Could you check a few things on this model? Use its own coordinates, in mm. A direction names the side the tool comes from. Round coordinates to 2 decimals unless told otherwise and drop trailing zeros. Write each loop counter-clockwise with the first axis right and the second up, starting at its lowest first coordinate (ties: lowest second). Pieces come first, ordered by that corner, then holes. Notation, with made-up numbers: (33, 73.25) -> (87, 73.25) arc R24 ccw to (87, 108.25) -> close; hole circle Ø5 at (36.25, -33). An arc over 180 degrees is marked (long way). Answer as CSV lines item,"result". Start each with the question number.
Q1. Imagine slicing it at D-D on z = 28.5. Please give me the cut outline in (x, y), and give its area (3 significant figures).
Q2. Imagine slicing it at C-C on x = -15. Please give me the cut outline in (y, z), and give its area (3 significant figures).
Q3. If I drill on line 1 (Y direction, x = 26, z = 9); line 2 (Y direction, x = -32.5, z = 38.5); line 3 (X direction, y = 37, z = 56), over which ranges is the centre line in solid material (lowest first)? Write a range as [from, to].
Q4. Will these pins go through, and if not, where does the flat tip stop? pin 1 Ø10 at (x, z) = (-39.5, 44.5) entering from -Y; pin 2 Ø8 at (x, z) = (-22, 10) entering from +Y; pin 3 Ø4 at (x, y) = (39.5, -3.5) entering from +Z.
Q5. Imagine slicing it at A-A on z = 49. Please give me the cut outline in (x, y).
Q6. Imagine slicing it at B-B on y = 22.5. Please give me the cut outline in (x, z).
Q7. If we mould it in two halves opening along Y, with no side actions, what happens to faces 4 (the flat face through (-27, -1, 63.5)), 5 (the flat face through (1, 29.04, 31)), 6 (the cylindrical face through (42.595, -4.481, 50.978))? For each: pulls with the +Y half, pulls with the -Y half, needs draft (parallel to the pull), parting line crosses it, or undercut.
Q8. For faces 1 (the flat face through (-34, -2, 38.1)), 2 (the cylindrical face through (0.95, 38.05, 40.91)), 3 (the flat face through (1, -33.137, 31)), which set-ups out of +Z, -Z, +X, -X, +Y, -Y let a thin tool reach every point of the face, with its end or its side?
from build123d import *

# Parameters (mm, degrees)
F0_W      = 108.688287437
F0_H      = 62.1764454991
F1_DEPTH  = 63.5
F2_R      = 6.35
F3_DEPTH  = 25.4
F4_W      = 45.188287437
F4_H      = 17.78
F4_H_2    = 62.1764454991
F5_DEPTH  = 25.4
F7_DEPTH  = 17.78
F9_DEPTH  = 97.7364454991
F11_DEPTH = 17.78
F13_DEPTH = 17.78


with BuildPart() as f1:
    # F0 (on Top) → F1 (new body)
    with BuildSketch(Plane.XY):
        with Locations((1.4459639788, -2.0484467968)):
            Rectangle(F0_W, F0_H)
    extrude(amount=F1_DEPTH)

    # F2 (on face) → F3 (cut)
    with BuildSketch(Plane.XY.offset(63.5)):
        with Locations((-33.8375324716, -2.0484467968)):
            Circle(F2_R)
        with Locations((36.7294604292, -2.0484467968)):
            Circle(F2_R)
    extrude(amount=-F3_DEPTH, mode=Mode.SUBTRACT)

    # F4 (on face) → F5 (join)
    with BuildSketch(Plane.XY.offset(63.5)):
        with Locations((1.4459639788, -42.0266695464)):
            Rectangle(F4_W, F4_H)
        with Locations((1.4459639788, -2.0484467968)):
            Rectangle(F4_W, F4_H_2)
        with Locations((1.4459639788, 37.9297759527)):
            Rectangle(F4_W, F4_H)
    extrude(amount=-F5_DEPTH)

    # F6 (on face) → F7 (cut, through all)
    with BuildSketch(Plane.XZ.offset(50.9166695464)):
        with BuildLine():
            ThreePointArc((24.0401076972, 63.5), (1.4459639788, 40.9058562815), (-21.1481797397, 63.5))
            Line((-21.1481797397, 63.5), (-21.1481797397, 38.1))
            Line((-21.1481797397, 38.1), (24.0401076972, 38.1))
            Line((24.0401076972, 38.1), (24.0401076972, 63.5))
        make_face()
    extrude(amount=-F7_DEPTH, mode=Mode.SUBTRACT)

    # F8 (on face) → F9 (cut, through all)
    with BuildSketch(Plane.XZ.offset(50.9166695464)):
        with BuildLine():
            Line((20.2301076972, 63.5), (-17.3381797397, 63.5))
            ThreePointArc((-17.3381797397, 63.5), (1.4459639788, 45.134926003), (20.2301076972, 63.5))
        make_face()
    extrude(amount=-F9_DEPTH, mode=Mode.SUBTRACT)

    # F10 (on face) → F11 (join, through all)
    with BuildSketch(Plane(origin=(0, 46.8197759527, 0), x_dir=(-1, 0, 0), z_dir=(0, 1, 0))):
        with BuildLine():
            ThreePointArc((21.1481797397, 63.5), (-1.4459639788, 40.9058562815), (-24.0401076972, 63.5))
            Line((-24.0401076972, 63.5), (-24.0401076972, 38.1))
            Line((-24.0401076972, 38.1), (21.1481797397, 38.1))
            Line((21.1481797397, 38.1), (21.1481797397, 63.5))
        make_face()
    extrude(amount=-F11_DEPTH)

    # F12 (on face) → F13 (cut, through all)
    with BuildSketch(Plane(origin=(0, 46.8197759527, 0), x_dir=(-1, 0, 0), z_dir=(0, 1, 0))):
        with BuildLine():
            ThreePointArc((21.1481797397, 63.5), (-1.4459639788, 40.9058562815), (-24.0401076972, 63.5))
            Line((-24.0401076972, 63.5), (-24.0401076972, 38.1))
            Line((-24.0401076972, 38.1), (21.1481797397, 38.1))
            Line((21.1481797397, 38.1), (21.1481797397, 63.5))
        make_face()
    extrude(amount=-F13_DEPTH, mode=Mode.SUBTRACT)


solid = f1.part
Checks:
1,outline,"(-52.9, -33.14) -> (55.79, -33.14) -> (55.79, 29.04) -> (-52.9, 29.04) -> close"
1,area,"6,760 mm^2"
2,outline,"(-50.92, 48.01) -> (-33.14, 48.01) -> (-33.14, 0) -> (29.04, 0) -> (29.04, 48.01) -> (46.82, 48.01) -> (46.82, 54.84) -> (-50.92, 54.84) -> close"
2,area,"3,650 mm^2"
3,line 1,"[-33.14, 29.04]"
3,line 2,"[-33.14, -8.26], [4.16, 29.04]"
3,line 3,"[-19.87, -15.59], [18.48, 22.76]"
4,pin 1,"y = -33.14"
4,pin 2,"y = 29.04"
4,pin 3,"z = 38.1"
5,outline,"(-52.9, -33.14) -> (-15.88, -33.14) -> (-15.88, -50.92) -> (-9.97, -50.92) -> (-9.97, 46.82) -> (-15.88, 46.82) -> (-15.88, 29.04) -> (-52.9, 29.04) -> close; (12.86, -50.92) -> (18.77, -50.92) -> (18.77, -33.14) -> (55.79, -33.14) -> (55.79, 29.04) -> (18.77, 29.04) -> (18.77, 46.82) -> (12.86, 46.82) -> close; hole circle Ø12.7 at (-33.84, -2.05); hole circle Ø12.7 at (36.73, -2.05)"
6,outline,"(-52.9, 0) -> (55.79, 0) -> (55.79, 63.5) -> (20.23, 63.5) arc R18.79 cw to (-17.34, 63.5) -> (-52.9, 63.5) -> close"
7,face 4,"needs draft"
7,face 5,"pulls with the +Y half"
7,face 6,"undercut"
8,face 1,"+Z"
8,face 2,"-Z, +Y"
8,face 3,"-Z, -Y"
